from build123d import *

# Parameters (mm, degrees)
ESTRUSIONE_ESTRUSIONE1_DEPTH = 30
SCHIZZO2_R                   = 2.25
TAGLIO_ESTRUSIONE1_DEPTH     = 3
SCHIZZO3_R                   = 1.75
TAGLIO_ESTRUSIONE2_DEPTH     = 3


with BuildPart() as part:
    # Schizzo1 → Estrusione-Estrusione1 (new body)
    with BuildSketch(Plane.XY):
        Polygon((0, 0), (-30, 0), (-30, 2), (-2, 2), (-2, 50), (0, 50), align=None)
    extrude(amount=ESTRUSIONE_ESTRUSIONE1_DEPTH)

    # Schizzo2 → Taglio-Estrusione1 (cut, through all)
    with BuildSketch(Plane.ZY.offset(2)):
        with Locations((15, 37)):
            Circle(SCHIZZO2_R)
        with Locations((15, 11.6)):
            Circle(SCHIZZO2_R)
    extrude(amount=-TAGLIO_ESTRUSIONE1_DEPTH, mode=Mode.SUBTRACT)

    # Schizzo3 → Taglio-Estrusione2 (cut, through all)
    with BuildSketch(Plane(origin=(0, 2, 0), x_dir=(1, 0, 0), z_dir=(0, 1, 0))):
        with Locations((-16, -15)):
            Circle(SCHIZZO3_R)
    extrude(amount=-TAGLIO_ESTRUSIONE2_DEPTH, mode=Mode.SUBTRACT)


solid = part.part
Design review of the part built by this model. Coordinates are the model's own, in mm. A direction names the side the tool comes from. Give positions to 0.01 mm unless a question says otherwise; leave off trailing zeros. Loops run counter-clockwise (first coordinate to the right, second up) from the corner with the lowest first, then second, coordinate; pieces in that order, holes last. Notation, with made-up numbers: M 2.5,85.5 L 20.5,85.5 A16 cw 20.5,104.5 Z; hole C -0.5,7.5 d6. An arc over 180 degrees is marked long. Write item = value, one per line.
Q1. We need section B-B (y = 11.6). Give the boundary of the cut face in (x, z).
Output values:
outline = M -2,0 L 0,0 L 0,12.75 L -2,12.75 Z; M -2,17.25 L 0,17.25 L 0,30 L -2,30 Z
Q2. We need section A-A (x = -16). Give the boundary of the cut face in (y, z), plus the area to 3 significant figures.
Output values:
outline = M 0,0 L 2,0 L 2,13.25 L 0,13.25 Z; M 0,16.75 L 2,16.75 L 2,30 L 0,30 Z
area = 53.0 mm^2
Q3. To check wall thickness, follow line 1 (Y direction, x = -0.9, z = 15); line 2 (Z direction, x = -16, y = 0.9); line 3 (X direction, y = 0.9, z = 15). State the ranges of each line that lie inside material, in increasing order. Write a range as [from, to].
Output values:
line_1 = [0, 9.35], [13.85, 34.75], [39.25, 50]
line_2 = [0, 13.25], [16.75, 30]
line_3 = [-30, -17.75], [-14.25, 0]
Q4. Insertion check: pin 1 (4 mm diameter, centred on y = 9, z = 21.5, fed in from +X); pin 2 (5.5 mm diameter, centred on x = -16, z = 15, fed in from +Y); pin 3 (15 mm diameter, centred on y = 31.5, z = 12, fed in from -X); pin 4 (10 mm diameter, centred on x = -11.5, y = 22, fed in from +Z). Each pin has a flat end and moves straight along its axis. Give the tip position at first contact, or say it passes through.
Output values:
pin_1 = 0
pin_2 = 2
pin_3 = -2
pin_4 = through
Q5. We need section D-D (z = 27.5). Give the boundary of the cut face in (x, y), plus the area to 3 significant figures.
Output values:
outline = M -30,0 L 0,0 L 0,50 L -2,50 L -2,2 L -30,2 Z
area = 156 mm^2
Q6. We need section C-C (z = 14). Give the boundary of the cut face in (x, y).
Output values:
outline = M -30,0 L -17.44,0 L -17.44,2 L -30,2 Z; M -14.56,0 L 0,0 L 0,9.58 L -2,9.58 L -2,2 L -14.56,2 Z; M -2,13.62 L 0,13.62 L 0,34.98 L -2,34.98 Z; M -2,39.02 L 0,39.02 L 0,50 L -2,50 Z
Q7. Draft analysis for pull direction Z (two halves, no side actions). For faces 3 (the cylindrical face through (-1.014, 38.897, 16.21)), 4 (the flat face through (-2, 26, 15)), 5 (the flat face through (-1.6, 17.7, 30)), state which applies: +Z half, -Z half, draft (parallel to the pull), parting line (faces both ways), or undercut.
Output values:
face_3 = undercut
face_4 = draft
face_5 = +Z half
Q8. For faces 1 (the flat face through (-30, 1, 15)), 2 (the flat face through (-13, 2, 15)), list the 3-axis set-ups (+Z, -Z, +X, -X, +Y, -Y) from which the entire face can be reached by the end or side of a thin tool; tool diameter is ignored.
Output values:
face_1 = +Z, -Z, -X, +Y, -Y
face_2 = +Z, -Z, -X, +Y
